Here's the drawing with two shaded views (mm, measured from the low corner). I have some questions. Round coordinates to 2 decimals unless told otherwise and drop trailing zeros. Loops run counter-clockwise (first coordinate to the right, second up) from the corner with the lowest first, then second, coordinate; pieces in that order, holes last. Notation, with made-up numbers: M -14,33.25 L 16,33.25 A33 cw 16,66.25 Z; hole C 46,76.5 d6. An arc over 180 degrees is marked long. Answer as CSV lines item,"result".
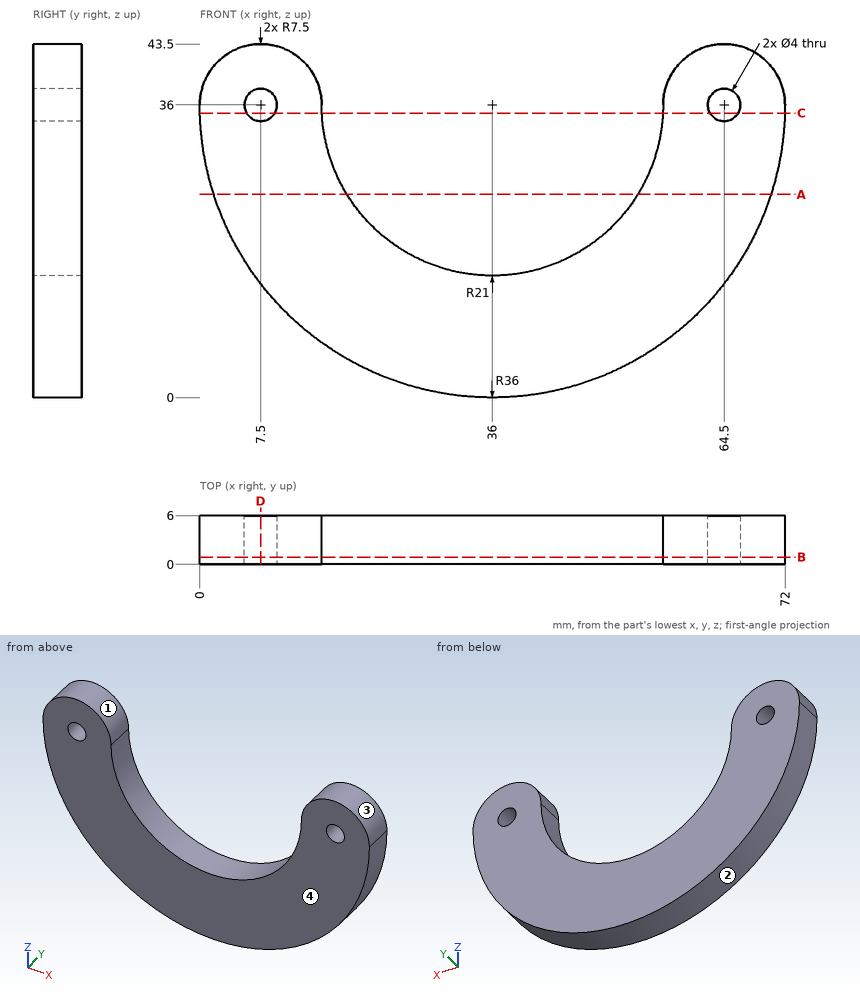
1. I want a section at D-D, the plane x = 7.5. Please give me the cut outline in (y, z), and give its area (3 significant figures).
Evaluation:
outline,"M 0,14.01 L 6,14.01 L 6,34 L 0,34 Z; M 0,38 L 6,38 L 6,43.5 L 0,43.5 Z"
area,"153 mm²"
2. I want a section at B-B, the plane y = 0.9. Please give me the cut outline in (x, z), and give its area (3 significant figures).
Evaluation:
outline,"M 0,36 A36 ccw 72,36 A7.5 ccw 57,36 A21 cw 15,36 A7.5 ccw Z; hole C 7.5,36 d4; hole C 64.5,36 d4"
area,"1,490 mm²"
3. I want a section at A-A, the plane z = 25. Please give me the cut outline in (x, y), and give its area (3 significant figures).
Evaluation:
outline,"M 1.72,0 L 18.11,0 L 18.11,6 L 1.72,6 Z; M 53.89,0 L 70.28,0 L 70.28,6 L 53.89,6 Z"
area,"197 mm²"
4. If I drill on line 1 (X direction, y = 3, z = 36); line 2 (X direction, y = 3.3, z = 35.5); line 3 (X direction, y = 5.6, z = 27), over which ranges is the centre line in solid material (lowest first)? Write a range as [from, to].
Evaluation:
line 1,"x = [0, 5.5], [9.5, 15], [57, 62.5], [66.5, 72]"
line 2,"x = [0, 5.56], [9.44, 15.01], [56.99, 62.56], [66.44, 72]"
line 3,"x = [1.14, 17.03], [54.97, 70.86]"
5. I want a section at C-C, the plane z = 35. Please give me the cut outline in (x, y), and give its area (3 significant figures).
Evaluation:
outline,"M 0.01,0 L 5.77,0 L 5.77,6 L 0.01,6 Z; M 9.23,0 L 15.02,0 L 15.02,6 L 9.23,6 Z; M 56.98,0 L 62.77,0 L 62.77,6 L 56.98,6 Z; M 66.23,0 L 71.99,0 L 71.99,6 L 66.23,6 Z"
area,"139 mm²"
6. We'd pull the mould along X, two halves only. Please class the marked faces 1, 2, 3 and 4: pulls with the +X half, pulls with the -X half, needs draft (parallel to the pull), parting line crosses it, or undercut.
Evaluation:
face 1,"undercut"
face 2,"parting line crosses it"
face 3,"undercut"
face 4,"needs draft"
